Can you work these out from the model? Positions are in its coordinate system, mm. A direction names the side the tool comes from. Give positions to 0.01 mm unless a question says otherwise; leave off trailing zeros. Write each loop counter-clockwise with the first axis right and the second up, starting at its lowest first coordinate (ties: lowest second). Pieces come first, ordered by that corner, then holes. Notation, with made-up numbers: (-35.5, -33.5) - (8.5, -33.5) arc R30 cw to (8.5, 5.5) - close; hole circle Ø8 at (-3, 15). An arc over 180 degrees is marked (long way). Return JSON: item names as keys, results as strings. Group by question number.
from build123d import *

# Parameters (mm, degrees)
SKETCH_1_R                      = 13
EXTRUDE_1_DEPTH                 = 42.8
SKETCH_2_R                      = 3.5
CUT_EXTRUDE_1_DEPTH             = 47.581541409
SKETCH_4_R                      = 1.6
CUT_EXTRUDE_2_DEPTH             = 47.581541409
EXTRUDE_2_DEPTH                 = 42.8
CUT_EXTRUDE_3_DEPTH             = 42.8
CUT_EXTRUDE_4_DEPTH             = 18.4
CUT_EXTRUDE_4_DEPTH_BACK        = 18.4
CUT_EXTRUDE_5_DEPTH             = 63.153760948
CUT_EXTRUDE_5_DEPTH_BACK        = 63.153760948
SKETCH_9_R                      = 1.5
CUT_EXTRUDE_6_DEPTH             = 63.153760948
CUT_EXTRUDE_6_DEPTH_BACK        = 1.5
SKETCH_10_R                     = 2.8
SKETCH_11_R                     = 2.8
CUT_EXTRUDE_7_DEPTH             = 1
CUT_EXTRUDE_8_REACH             = 47.874
CUT_EXTRUDE_8_DIRECTION_2_REACH = 47.874
CUT_EXTRUDE_9_DEPTH             = 59.977453319
CUT_EXTRUDE_10_DEPTH            = 59.977453319


with BuildPart() as part:
    # 草图1 → 凸台-拉伸1 (new body)
    with BuildSketch(Plane.XY):
        Circle(SKETCH_1_R)
    extrude(amount=EXTRUDE_1_DEPTH)

    # 草图2 → 切除-拉伸1 (cut, through all)
    with BuildSketch(Plane.XY.offset(42.8)):
        Circle(SKETCH_2_R)
    extrude(amount=-CUT_EXTRUDE_1_DEPTH, mode=Mode.SUBTRACT)

    # 草图4 → 切除-拉伸2 (cut, through all)
    with BuildSketch(Plane(origin=(0, 0, 0), x_dir=(-1, 0, 0), z_dir=(0, 0, -1))):
        with Locations((0, 7)):
            Circle(SKETCH_4_R)
        with Locations((7, 0)):
            Circle(SKETCH_4_R)
        with Locations((0, -7)):
            Circle(SKETCH_4_R)
        with Locations((-7, 0)):
            Circle(SKETCH_4_R)
    extrude(amount=-CUT_EXTRUDE_2_DEPTH, mode=Mode.SUBTRACT)

    # 草图5 → 凸台-拉伸2 (add)
    with BuildSketch(Plane(origin=(0, 0, 0), x_dir=(-1, 0, 0), z_dir=(0, 0, -1))):
        with BuildLine():
            ThreePointArc((-12.755, -2.511966361), (-17.099037385, -9.686319722), (-25, -12.5))
            Line((-25, -12.5), (-37.5, -12.5))
            Line((-37.5, -12.5), (-37.5, -15.5))
            Line((-37.5, -15.5), (22.5, -15.5))
            Line((22.5, -15.5), (22.5, -12.5))
            ThreePointArc((22.5, -12.5), (16.150397643, -8.956340583), (12.751851852, -2.527899197))
            ThreePointArc((12.751851852, -2.527899197), (-0.008120438, -12.999997464), (-12.755, -2.511966361))
        make_face()
    extrude(amount=-EXTRUDE_2_DEPTH)

    # 草图7 → 切除-拉伸3 (cut)
    with BuildSketch(Plane(origin=(0, 0, 0), x_dir=(-1, 0, 0), z_dir=(0, 0, -1))):
        with BuildLine():
            ThreePointArc((12.5, 0), (0, 12.5), (-12.5, 0))
            ThreePointArc((-12.5, 0), (-12.563913397, -1.262438117), (-12.755, -2.511966361))
            ThreePointArc((-12.755, -2.511966361), (0.008120438, 12.999997464), (12.751851852, -2.527899197))
            ThreePointArc((12.751851852, -2.527899197), (12.563118434, -1.270207041), (12.5, 0))
        make_face()
    extrude(amount=-CUT_EXTRUDE_3_DEPTH, mode=Mode.SUBTRACT)

    # 草图8 → 切除-拉伸4 (cut, two sides: drawn at the far end of the back side and taken through both)
    with BuildSketch(Plane.XY.offset(21.4).offset(-CUT_EXTRUDE_4_DEPTH_BACK)):
        with BuildLine():
            ThreePointArc((-12.5, 0), (-8.838834765, -8.838834765), (0, -12.5))
            ThreePointArc((0, -12.5), (8.838834765, -8.838834765), (12.5, 0))
            ThreePointArc((12.5, 0), (0, 12.5), (-12.5, 0))
        make_face()
        with BuildLine():
            Line((-22.5, -12.5), (0, -12.5))
            ThreePointArc((0, -12.5), (-8.838834765, -8.838834765), (-12.5, 0))
            ThreePointArc((-12.5, 0), (-15.307618379, -8.003905297), (-22.5, -12.5))
        make_face()
        with BuildLine():
            ThreePointArc((12.5, 0), (8.838834765, -8.838834765), (0, -12.5))
            Line((0, -12.5), (25, -12.5))
            ThreePointArc((25, -12.5), (16.161165235, -8.838834765), (12.5, 0))
        make_face()
    extrude(amount=CUT_EXTRUDE_4_DEPTH + CUT_EXTRUDE_4_DEPTH_BACK, mode=Mode.SUBTRACT)

    # 草图9 → 切除-拉伸5 (cut, two sides: drawn at the far end of the back side and taken through both)
    with BuildSketch(Plane(origin=(0, -12.5, 0), x_dir=(1, 0, 0), z_dir=(0, 1, 0)).offset(-CUT_EXTRUDE_5_DEPTH_BACK)):
        with Locations(Location((32.5, -13.9, 0), (0, 0, 180))):
            Circle(SKETCH_9_R)
        with Locations(Location((32.5, -28.9, 0), (0, 0, 180))):
            Circle(SKETCH_9_R)
        with Locations(Location((-17.5, -13.9, 0), (0, 0, 180))):
            Circle(SKETCH_9_R)
        with Locations(Location((-17.5, -28.9, 0), (0, 0, 180))):
            Circle(SKETCH_9_R)
    extrude(amount=CUT_EXTRUDE_5_DEPTH + CUT_EXTRUDE_5_DEPTH_BACK, mode=Mode.SUBTRACT)

    # 草图10 → 切除-拉伸6 (cut, two sides: drawn at the far end of the back side and taken through both)
    with BuildSketch(Plane(origin=(0, -12.5, 0), x_dir=(1, 0, 0), z_dir=(0, 1, 0)).offset(-CUT_EXTRUDE_6_DEPTH_BACK)):
        with Locations(Location((-17.5, -13.9, 0), (0, 0, 180))):
            Circle(SKETCH_10_R)
        with Locations(Location((-17.5, -28.9, 0), (0, 0, 180))):
            Circle(SKETCH_10_R)
        with Locations(Location((32.5, -13.9, 0), (0, 0, 180))):
            Circle(SKETCH_10_R)
        with Locations(Location((32.5, -28.9, 0), (0, 0, 180))):
            Circle(SKETCH_10_R)
    extrude(amount=CUT_EXTRUDE_6_DEPTH + CUT_EXTRUDE_6_DEPTH_BACK, mode=Mode.SUBTRACT)

    # 草图11 → 切除-拉伸7 (cut)
    with BuildSketch(Plane(origin=(0, 0, 0), x_dir=(-1, 0, 0), z_dir=(0, 0, -1))):
        with Locations((0, 7)):
            Circle(SKETCH_11_R)
        with Locations((7, 0)):
            Circle(SKETCH_11_R)
        with Locations((0, -7)):
            Circle(SKETCH_11_R)
        with Locations((-7, 0)):
            Circle(SKETCH_11_R)
    cut_extrude_7 = extrude(amount=-CUT_EXTRUDE_7_DEPTH, mode=Mode.SUBTRACT)

    # 镜向1: 切除-拉伸7 across plane
    add(cut_extrude_7.mirror(Plane.XY.offset(21.4)), mode=Mode.SUBTRACT)

    # 切除-拉伸8: up to this face of the body (flat: up to its plane)
    cut_extrude_8_end = Plane(part.part.faces().sort_by_distance((0, 11.963227236, 3))[0])
    # 草图12 → 切除-拉伸8 (cut, up to the picked face)
    with BuildSketch(Plane.XY.offset(21.4), mode=Mode.PRIVATE) as cut_extrude_8_sk1:
        with BuildLine():
            Line((8.291561976, -12.5), (-8.291561976, -12.5))
            ThreePointArc((-8.291561976, -12.5), (0, -15), (8.291561976, -12.5))
        make_face()
    cut_extrude_8_tool1 = split(extrude(cut_extrude_8_sk1.sketch, amount=-CUT_EXTRUDE_8_REACH, mode=Mode.PRIVATE), bisect_by=cut_extrude_8_end, keep=Keep.BOTH, mode=Mode.PRIVATE)
    add(cut_extrude_8_tool1.solids().sort_by(Axis((0, -13.507506, 21.4), (0, 0, -1)))[0], mode=Mode.SUBTRACT)

    # 切除-拉伸8 direction 2: up to this face of the body (flat: up to its plane)
    cut_extrude_8_direction_2_end = Plane(part.part.faces().sort_by_distance((0, 11.963227236, 39.8))[0])
    # 草图12 → 切除-拉伸8 direction 2 (cut, up to the picked face)
    with BuildSketch(Plane.XY.offset(21.4), mode=Mode.PRIVATE) as cut_extrude_8_direction_2_sk1:
        with BuildLine():
            Line((8.291561976, -12.5), (-8.291561976, -12.5))
            ThreePointArc((-8.291561976, -12.5), (0, -15), (8.291561976, -12.5))
        make_face()
    cut_extrude_8_direction_2_tool1 = split(extrude(cut_extrude_8_direction_2_sk1.sketch, amount=CUT_EXTRUDE_8_DIRECTION_2_REACH, mode=Mode.PRIVATE), bisect_by=cut_extrude_8_direction_2_end, keep=Keep.BOTH, mode=Mode.PRIVATE)
    add(cut_extrude_8_direction_2_tool1.solids().sort_by(Axis((0, -13.507506, 21.4), (0, 0, 1)))[0], mode=Mode.SUBTRACT)

    # 草图13 → 切除-拉伸9 (cut, through all)
    with BuildSketch(Plane(origin=(0, 0, 0), x_dir=(-1, 0, 0), z_dir=(0, 0, -1))):
        with BuildLine():
            ThreePointArc((10.98532184, 5.964285714), (0, 11), (-10.98532184, 5.964285714))
            ThreePointArc((-10.98532184, 5.964285714), (0, 12.5), (10.98532184, 5.964285714))
        make_face()
    extrude(amount=-CUT_EXTRUDE_9_DEPTH, mode=Mode.SUBTRACT)

    # 草图14 → 切除-拉伸10 (cut, through all)
    with BuildSketch(Plane.XY.offset(42.8)):
        with BuildLine():
            ThreePointArc((-21.180750885, -12.128017377), (-20.029150419, -12.406420537), (-18.848076825, -12.5))
            ThreePointArc((-18.848076825, -12.5), (-13.544775966, -10.303300859), (-11.348076825, -5))
            ThreePointArc((-11.348076825, -5), (-11.411025921, -4.030322808), (-11.59881652, -3.076923029))
            ThreePointArc((-11.59881652, -3.076923029), (-11.98420936, -1.977199407), (-12.535301413, -0.950448592))
            ThreePointArc((-12.535301413, -0.950448592), (-15.17777558, -7.838846674), (-21.180750885, -12.128017377))
        make_face()
        with BuildLine():
            ThreePointArc((-12.535301413, -0.950448592), (-24.780598437, -0.411406825), (-21.180750885, -12.128017377))
            ThreePointArc((-21.180750885, -12.128017377), (-15.17777558, -7.838846674), (-12.535301413, -0.950448592))
        make_face()
        with BuildLine():
            ThreePointArc((-12.5, 0), (-12.508828395, -0.475551973), (-12.535301413, -0.950448592))
            ThreePointArc((-12.535301413, -0.950448592), (-11.98420936, -1.977199407), (-11.59881652, -3.076923029))
            ThreePointArc((-11.59881652, -3.076923029), (-11.71218701, 2.61240798), (-9.19183311, 7.714285714))
            ThreePointArc((-9.19183311, 7.714285714), (-10.126451524, 6.87810096), (-10.98532184, 5.964285714))
            ThreePointArc((-10.98532184, 5.964285714), (-12.115414211, 3.076806543), (-12.5, 0))
        make_face()
        with BuildLine():
            ThreePointArc((-21.180750885, -12.128017377), (-21.835397512, -12.331663089), (-22.5, -12.5))
            Line((-22.5, -12.5), (-18.848076825, -12.5))
            ThreePointArc((-18.848076825, -12.5), (-20.029150419, -12.406420537), (-21.180750885, -12.128017377))
        make_face()
        with BuildLine():
            ThreePointArc((21.931346237, -12.117481755), (20.724136458, -12.403791939), (19.48717527, -12.5))
            Line((19.48717527, -12.5), (25, -12.5))
            ThreePointArc((25, -12.5), (23.453798515, -12.404001813), (21.931346237, -12.117481755))
        make_face()
        with BuildLine():
            ThreePointArc((11.692305187, -2.699999893), (13.226184899, -9.479959796), (19.48717527, -12.5))
            ThreePointArc((19.48717527, -12.5), (20.724136458, -12.403791939), (21.931346237, -12.117481755))
            ThreePointArc((21.931346237, -12.117481755), (15.316506899, -7.904426694), (12.513458103, -0.579889175))
            ThreePointArc((12.513458103, -0.579889175), (12.027181322, -1.610624584), (11.692305187, -2.699999893))
        make_face()
        with BuildLine():
            ThreePointArc((12.513458103, -0.579889175), (15.316506899, -7.904426694), (21.931346237, -12.117481755))
            ThreePointArc((21.931346237, -12.117481755), (25.950663791, -9.214161233), (27.48717527, -4.5))
            ThreePointArc((27.48717527, -4.5), (21.513287639, 3.239177519), (12.513458103, -0.579889175))
        make_face()
        with BuildLine():
            ThreePointArc((12, 0), (11.922828151, -1.358737973), (11.692305187, -2.699999893))
            ThreePointArc((11.692305187, -2.699999893), (12.027181322, -1.610624584), (12.513458103, -0.579889175))
            ThreePointArc((12.513458103, -0.579889175), (12.503364979, -0.290022661), (12.5, 0))
            ThreePointArc((12.5, 0), (12.115414211, 3.076806543), (10.98532184, 5.964285714))
            ThreePointArc((10.98532184, 5.964285714), (10.126451524, 6.87810096), (9.19183311, 7.714285714))
            ThreePointArc((9.19183311, 7.714285714), (11.276125162, 4.104753506), (12, 0))
        make_face()
    extrude(amount=-CUT_EXTRUDE_10_DEPTH, mode=Mode.SUBTRACT)


solid = part.part
1) I need wall thicknesses on line 1 along Y through (x, z) = (0, 1.7); line 2 along Z through (x, y) = (-17.5, -15); line 3 along Z through (x, y) = (3, 9.25). Which ranges of each line are inside material? Lowest first, please.
2) Imagine slicing it at C-C, the plane x = -18. Write out the boundary of the cut face in (y, z) (3 decimals).
3) Imagine slicing it at A-A, the plane z = 28.9. Write out the boundary of the cut face in (x, y).
4) Will these pins go through, and if not, where does the flat tip stop? pin 1 Ø3.5 at (x, y) = (-7, 0) entering from -Z; pin 2 Ø4.5 at (x, z) = (-17, 16) entering from +Y; pin 3 Ø4 at (x, z) = (-17.5, 13.9) entering from +Y.
5) On a 3-axis mill with a long thin cutter (end or side, diameter ignored), from which of +Z, -Z, +X, -X, +Y, -Y can I reach the whole of each face in a straight line? I mean faces 5 (the face through (-15.278, -13.26, 27.196)), 6 (the face through (-9, 0, 41.8)), 7 (the face through (-5.4, 0.07, 1.99)), 8 (the face through (0.607, -9.733, 0.493)), 9 (the face through (-16, -14.76, 28.97)). Say none if no direction works.
6) We'd pull the mould along X, two halves only. Please class faces 1 (the face through (13.164, -9.401, 41.321)), 2 (the face through (-22.5, -14, 21)), 3 (the face through (34.722, -13.26, 12.196)), 4 (the face through (-15, -12.5, 22)): pulls with the +X half, pulls with the -X half, needs draft (parallel to the pull), parting line crosses it, or undercut.
7) Imagine slicing it at B-B, the plane y = -10.5. Write out the boundary of the cut face in (x, z).
8) Imagine slicing it at D-D, the plane y = -7. Write out the boundary of the cut face in (x, z).
Resolved:
{
 "1": {"line 1": "-15.5 to -8.6, -5.4 to -3.5, 3.5 to 5.4, 8.6 to 11", "line 2": "0 to 12.4, 15.4 to 27.4, 30.4 to 42.8", "line 3": "0 to 3, 39.8 to 42.8"},
 "2": {"outline": "(-15.5, 0) - (-12.452, 0) - (-12.452, 3) - (-12.5, 3) - (-12.5, 11.145) - (-14, 11.145) - (-14, 12.486) - (-15.5, 12.486) - close; (-15.5, 15.314) - (-14, 15.314) - (-14, 16.655) - (-12.5, 16.655) - (-12.5, 26.145) - (-14, 26.145) - (-14, 27.486) - (-15.5, 27.486) - close; (-15.5, 30.314) - (-14, 30.314) - (-14, 31.655) - (-12.5, 31.655) - (-12.5, 39.8) - (-12.452, 39.8) - (-12.452, 42.8) - (-15.5, 42.8) - close"},
 "3": {"outline": "(-22.5, -15.5) - (-19, -15.5) - (-19, -14) - (-20.3, -14) - (-20.3, -12.5) - (-22.5, -12.5) - close; (-16, -15.5) - (31, -15.5) - (31, -14) - (29.7, -14) - (29.7, -12.5) - (8.29, -12.5) arc R15 cw to (-8.29, -12.5) - (-14.7, -12.5) - (-14.7, -14) - (-16, -14) - close; (34, -15.5) - (37.5, -15.5) - (37.5, -12.5) - (35.3, -12.5) - (35.3, -14) - (34, -14) - close"},
 "4": {"pin 1": "z = 1", "pin 2": "y = -12.5", "pin 3": "y = -14"},
 "5": {"face 5": "+Y", "face 6": "+Z", "face 7": "+Z, -Z", "face 8": "-Z", "face 9": "+Y, -Y"},
 "6": {"face 1": "pulls with the +X half", "face 2": "pulls with the -X half", "face 3": "undercut", "face 4": "needs draft"},
 "7": {"outline": "(-13.75, 0) - (14.2, 0) - (14.2, 3) - (-13.75, 3) - close; (-13.75, 39.8) - (14.2, 39.8) - (14.2, 42.8) - (-13.75, 42.8) - close"},
 "8": {"outline": "(-11.62, 0) - (-2.8, 0) - (-2.8, 1) - (-1.6, 1) - (-1.6, 3) - (-11.62, 3) - close; (-11.62, 39.8) - (-1.6, 39.8) - (-1.6, 41.8) - (-2.8, 41.8) - (-2.8, 42.8) - (-11.62, 42.8) - close; (1.6, 1) - (2.8, 1) - (2.8, 0) - (11.89, 0) - (11.89, 3) - (1.6, 3) - close; (1.6, 39.8) - (11.89, 39.8) - (11.89, 42.8) - (2.8, 42.8) - (2.8, 41.8) - (1.6, 41.8) - close"}
}
